Read the model definition and answer for the solid it produces. Units are mm, in the model's axes. A direction names the side the tool comes from. Coordinates: 2 decimals unless noted, no trailing zeros. Write each loop counter-clockwise with the first axis right and the second up, starting at its lowest first coordinate (ties: lowest second). Pieces come first, ordered by that corner, then holes. Notation, with made-up numbers: (-27.5, -9.5) -> (-14.5, -9.5) arc R25 ccw to (-14.5, 22.5) -> close; hole circle Ø3 at (75, -8.5). An arc over 180 degrees is marked (long way). Answer as a JSON object with one key per item and string values. Group by question number.
(1) Straight lines are drawn through the part: L1, parallel to X at y = 0, z = 14.45; L2, parallel to Z at x = 2.5, y = 1.5. For each, find the intervals that lie inside material, in ascending order.
(2) Find section B-B (z = -33). Give the vertices of the cut face in (x, y), then the cut area to 3 significant figures.
(3) For a pull along Y with two mould halves and no side action, classify faces 1 (the face through (10.5, -10.4, 4.9)), 2 (the face through (0, 0, 11)), 3 (the face through (4.88, -1.08, -31.27)) as +Y half, -Y half, draft (parallel to the pull), parting line (faces both ways), or undercut.
(4) Which of the six approach directions +Z, -Z, +X, -X, +Y, -Y give full straight-line access (tool end or side, diameter ignored) to faces 4 (the face through (-2.17, 9.76, 12.96)), 5 (the face through (0, -12.5, 5))?
(5) Find section A-A (z = 7.5). Give the vertices of the cut face in (x, y), then the cut area to 3 significant figures.
(6) Flat-ended cylindrical pins translate along their axes: P1, Ø3, axis at y = 0, z = -3.5, coming from the -X side; P2, Ø10, axis at x = 4, z = -24, coming from the +Y side; P3, Ø6, axis at y = -3, z = -31.5, coming from the +X side. Find the tip coordinate at first contact, or state that the pin passes through.
Autodesk Fusion 360 part; units mm, degrees
sketch "Sketch1" plane through (0, 0, 0) normal (0, 0, 1) x (1, 0, 0)
  circle A0 centre (0, 0) radius 7.5
  line L0 (-5.5, 12.5) -> (5.5, 12.5)
  line L1 (12.5, 5.5) -> (12.5, -5.5)
  line L2 (5.5, -12.5) -> (-5.5, -12.5)
  line L3 (-12.5, -5.5) -> (-12.5, 5.5)
  circle A1 centre (0, 0) radius 10
  arc A2 (-5.5, 12.5) -> (-12.5, 5.5) centre (-5.5, 5.5) ccw
  arc A3 (12.5, 5.5) -> (5.5, 12.5) centre (5.5, 5.5) ccw
  arc A4 (5.5, -12.5) -> (12.5, -5.5) centre (5.5, -5.5) ccw
  arc A5 (-12.5, -5.5) -> (-5.5, -12.5) centre (-5.5, -5.5) ccw
  line L4 (-10.4497, 10.4497) -> (10.4497, -10.4497)
  line L5 (10.4497, 10.4497) -> (0, 0)
  point P0 (-12.5, 12.5)
  dimension "d1" = 15
  dimension "d2" = 20
  dimension "d5" = 7
extrude "Extrude1" add sketch "Sketch1" along normal blind 10 contours L1 A1 A3 A4 L4 L5 | L0 A1 A2 A3 L4 L5 | L2 L3 A1 A2 A4 A5 L4 makes body 1
extrude "Extrude2" add sketch "Sketch1" along normal blind 16 contours A0 A1 L4 L5 | A0 A1 L4 L5 | A0 A1 L4 bodies 1
extrude "Extrude3" add sketch "Sketch1" along normal blind 11 contours A0 L4 L5 | A0 L4 L5 | A0 L4 bodies 1
sketch "Sketch2" plane through (0, 0, 0) normal (1, 0, 0) x (0, 0, -1)
  line L0 (14.0161, 0) -> (49.0161, 0)
  line L1 (49.0161, 0) -> (49.0161, 5)
  line L2 (49.0161, 5) -> (14.0161, 5)
  line L3 (14.0161, 5) -> (14.0161, 0)
  dimension "d12" = 35
  dimension "d13" = 5
revolve "Revolve1" add sketch "Sketch2" angle 360 about axis through (0, 0, -14.0161) along (0, 0, -1) separate body makes body 2
sketch "Sketch3" plane through (0, 0, 0) normal (0, 0, -1) x (-1, 0, 0)
  arc A0 (12.5, 5.5) -> (5.5, 12.5) centre (5.5, 5.5) ccw
  line L0 (5.5, 12.5) -> (-5.5, 12.5)
  arc A1 (-5.5, 12.5) -> (-12.5, 5.5) centre (-5.5, 5.5) ccw
  line L1 (-12.5, 5.5) -> (-12.5, -5.5)
  arc A2 (-12.5, -5.5) -> (-5.5, -12.5) centre (-5.5, -5.5) ccw
  line L2 (-5.5, -12.5) -> (5.5, -12.5)
  arc A3 (5.5, -12.5) -> (12.5, -5.5) centre (5.5, -5.5) ccw
  line L3 (12.5, -5.5) -> (12.5, 5.5)
  line L4 (-11.5, 5) -> (11.5, 5)
  line L5 (11.5, -5) -> (-11.5, -5)
  line L6 (-12.5, -4) -> (-12.5, 4)
  arc A4 (-11.5, 5) -> (-12.5, 4) centre (-11.5, 4) ccw
  arc A5 (-12.5, -4) -> (-11.5, -5) centre (-11.5, -4) ccw
  line L7 (-12.5, 0) -> (17.5, 0) construction
  line L8 (12.5, 4) -> (12.5, -4)
  arc A6 (12.5, 4) -> (11.5, 5) centre (11.5, 4) ccw
  arc A7 (11.5, -5) -> (12.5, -4) centre (11.5, -4) ccw
  point P0 (-12.5, 5)
  point P1 (-12.5, -5)
  dimension "d15" = 10
  dimension "d16" = 1
  dimension "d17" = 1
loft "Loft1" add profiles "Sketch3" section 1 contours L1 L3 L4 L5 L6 A4 A5 L8 A6 A7 section 2 face at (-1.5459, -1.0946, -14.0161) on bodies 2 bodies 2 1
Results below:
{
 "1": {"L1": "x = -10 to -7.5, 7.5 to 10", "L2": "z = -49.02 to 11"},
 "2": {"outline": "circle Ø10 at (0, 0)", "area": "78.5 mm2"},
 "3": {"face 1": "-Y half", "face 2": "undercut", "face 3": "parting line"},
 "4": {"face 4": "+Z", "face 5": "+Z, -Z, +X, -X, -Y"},
 "5": {"outline": "(-12.5, -5.5) arc R7 ccw to (-5.5, -12.5) -> (5.5, -12.5) arc R7 ccw to (12.5, -5.5) -> (12.5, 5.5) arc R7 ccw to (5.5, 12.5) -> (-5.5, 12.5) arc R7 ccw to (-12.5, 5.5) -> close", "area": "583 mm2"},
 "6": {"P1": "stops at x = -11.43", "P2": "stops at y = 5", "P3": "stops at x = 5"}
}
